Build history of the part. All positions in model axes, mm. A direction names the side the tool comes from. Round coordinates to 2 decimals unless told otherwise and drop trailing zeros. Loops run counter-clockwise (first coordinate to the right, second up) from the corner with the lowest first, then second, coordinate; pieces in that order, holes last.
from build123d import *

# Parameters (mm, degrees)
SKETCH1_R            = 8.9
BOSS_EXTRUDE1_DEPTH  = 30
SKETCH2_W            = 24
SKETCH2_H            = 23.8
CUT_EXTRUDE1_DEPTH   = 82.46195431
M3_CLEARANCE_HOLE1_D = 3.4
SKETCH4_W            = 3
SKETCH4_H            = 6
CUT_EXTRUDE2_DEPTH   = 6.19


with BuildPart() as part:
    # Sketch1 → Boss-Extrude1 (new body)
    with BuildSketch(Plane(origin=(0, 0, 0), x_dir=(0, 0, -1), z_dir=(1, 0, 0))):
        with BuildLine():
            Line((0, 11.9), (60, 11.9))
            ThreePointArc((60, 11.9), (71.9, 0), (60, -11.9))
            Line((60, -11.9), (0, -11.9))
            ThreePointArc((0, -11.9), (-11.9, 0), (0, 11.9))
        make_face()
        Circle(SKETCH1_R, mode=Mode.SUBTRACT)
        with Locations(Location((60, 0, 0), (0, 0, 180))):
            Circle(SKETCH1_R, mode=Mode.SUBTRACT)
    extrude(amount=BOSS_EXTRUDE1_DEPTH)

    # Sketch2 → Cut-Extrude1 (cut, through all)
    with BuildSketch(Plane(origin=(0, 11.9, 0), x_dir=(1, 0, 0), z_dir=(0, 1, 0))):
        with Locations((15, 0)):
            Rectangle(SKETCH2_W, SKETCH2_H)
        with Locations((15, 60)):
            Rectangle(SKETCH2_W, SKETCH2_H)
    extrude(amount=-CUT_EXTRUDE1_DEPTH, mode=Mode.SUBTRACT)

    # M3 Clearance Hole1 (through all)
    with Locations(Plane(origin=(30, -5.9, -15.34), x_dir=(0, 0, 1), z_dir=(1, 0, 0))):
        with Locations((0, 0), (0, -11.8), (-29.32, -11.8), (-29.32, 0)):
            Hole(M3_CLEARANCE_HOLE1_D / 2)

    # Sketch4 → Cut-Extrude2 (cut)
    with BuildSketch(Plane(origin=(0, 0, -48.1), x_dir=(-1, 0, 0), z_dir=(0, 0, -1))):
        with Locations((-21.5, -5.9)):
            Rectangle(SKETCH4_W, SKETCH4_H)
        with Locations((-21.5, 5.9)):
            Rectangle(SKETCH4_W, SKETCH4_H)
        with Locations((-8.5, -5.9)):
            Rectangle(SKETCH4_W, SKETCH4_H)
        with Locations((-8.5, 5.9)):
            Rectangle(SKETCH4_W, SKETCH4_H)
    cut_extrude2 = extrude(amount=-CUT_EXTRUDE2_DEPTH, mode=Mode.SUBTRACT)

    # Mirror1: Cut-Extrude2 across plane
    add(cut_extrude2.mirror(Plane.XY.offset(-30)), mode=Mode.SUBTRACT)


solid = part.part
(1) Slice it at C-C on x = 21.5. List the corners of the cut face in (y, z).
Responses:
outline: (-11.9, -48.1) - (-8.9, -48.1) - (-8.9, -41.91) - (-2.9, -41.91) - (-2.9, -48.1) - (2.9, -48.1) - (2.9, -41.91) - (8.9, -41.91) - (8.9, -48.1) - (11.9, -48.1) - (11.9, -11.9) - (8.9, -11.9) - (8.9, -18.09) - (2.9, -18.09) - (2.9, -11.9) - (-2.9, -11.9) - (-2.9, -18.09) - (-8.9, -18.09) - (-8.9, -11.9) - (-11.9, -11.9) - close
(2) Which spindle directions (+Z, -Z, +X, -X, +Y, -Y) get a long thin tool onto all of the face, cutting with end or side? Do faces 4 (the face through (10, 5.2, -46.4)), 5 (the face through (22, 6, -18.09)), 6 (the face through (27, -5, -52)). Say none if no direction does.
Responses:
face 4: -Z
face 5: +Z
face 6: -Z, +Y, -Y
(3) Slice it at B-B on x = 17. List the corners of the cut face in (y, z), plus the area to 3 significant figures.
Responses:
outline: (-11.9, -48.1) - (11.9, -48.1) - (11.9, -11.9) - (-11.9, -11.9) - close; hole circle Ø3.4 at (-5.9, -44.66); hole circle Ø3.4 at (-5.9, -15.34); hole circle Ø3.4 at (5.9, -44.66); hole circle Ø3.4 at (5.9, -15.34)
area: 825 mm2
(4) Slice it at D-D on z = -44.66. Count the separate pieces of the cut face and the enclosed holes in it, plus the area to 3 significant figures.
Responses:
separate pieces: 3
enclosed holes: 0
area: 479 mm2
(5) Pull direction Y, two halves, no side cores. Call faces 1 (the face through (30, 0, -31)), 2 (the face through (1.479, 0.262, -71.897)), 3 (the face through (23, -6.6, -46.4)): +Y half, -Y half, draft (parallel to the pull), parting line (faces both ways), or undercut.
Responses:
face 1: draft
face 2: parting line
face 3: undercut
(6) Pin check, flat tips, straight feed: P1, Ø7, axis at x = 11.5, y = -4.5, coming from the +Z side; P2, Ø4, axis at y = -1.5, z = -18.5, coming from the -X side; P3, Ø2.5, axis at x = 21, y = 5, coming from the -Z side; P4, Ø0.9, axis at x = 21.5, y = -5, coming from the -Z side. Stop position of each tip, or through.
Responses:
P1: stops at z = -11.9
P2: stops at x = 0
P3: stops at z = -48.1
P4: stops at z = -41.91
(7) Slice it at A-A on z = -10. List the corners of the cut face in (x, y), plus the area to 3 significant figures.
Responses:
outline: (0, -11.9) - (3, -11.9) - (3, 11.9) - (0, 11.9) - close; (27, -11.9) - (30, -11.9) - (30, 11.9) - (27, 11.9) - close
area: 143 mm2
(8) Probe line 1 (Y direction, x = 4.5, z = -15.34); line 2 (X direction, y = 8, z = -46.5); line 3 (Z direction, x = 25, y = 5.9). List the from-to ranges inside material, lowest first.
Responses:
line 1: y = -11.9 to -7.6, -4.2 to 4.2, 7.6 to 11.9
line 2: x = 0 to 7, 10 to 20, 23 to 30
line 3: z = -48.1 to -46.36, -42.96 to -17.04, -13.64 to -11.9
